The drawing under review shows one solid part. Ordinate dimensions are in mm from its lowest x, y, z. A direction names the side the tool comes from. Coordinates: 2 decimals unless noted, no trailing zeros. Write each loop counter-clockwise with the first axis right and the second up, starting at its lowest first coordinate (ties: lowest second). Pieces come first, ordered by that corner, then holes. Notation, with made-up numbers: (24, -32.5) - (53, -32.5) arc R5 ccw to (53, -26.5) - close; hole circle Ø10 at (85, 50). An arc over 180 degrees is marked (long way). Put each result on its own line as item: value. Start each with the question number.
Item 1: Mouldability with a two-part tool opening along Y and no side actions: class the marked faces 1, 2 and 3 as pulls with the +Y half, pulls with the -Y half, needs draft (parallel to the pull), parting line crosses it, or undercut.
Item 2: Consider section A-A on x = 77.5. Give the boundary of the cut face in (y, z).
Item 3: Machinability: for the marked faces 4 and 5, which of the approach directions +Z, -Z, +X, -X, +Y, -Y give a long, thin tool a straight path to every point of the face, cutting with its end or side? Answer none if there is none.
Item 4: To check wall thickness, follow L1, parallel to Y at x = 35.5, z = 16.5; L2, parallel to Z at x = 56.2, y = 2.1; L3, parallel to X at y = 10, z = 32.5. State the ranges of each line that lie inside material, in increasing order. Write a range as [from, to].
Item 5: Consider section D-D on z = 47.5. Give the boundary of the cut face in (x, y), then the cut area to 3 significant figures.
Item 6: Consider section C-C on x = 56.2. Give the boundary of the cut face in (y, z), then the cut area to 3 significant figures.
Item 7: For pin 1 (12 mm diameter, centred on y = 6, z = 38, fed in from +X); pin 2 (11 mm diameter, centred on x = 56.2, z = 25, fed in from -Y), all flat-tipped, find the tip position at first contact; note any pin that passes through.
Item 8: Consider section B-B on z = 25. Give the boundary of the cut face in (x, y), then the cut area to 3 significant figures.
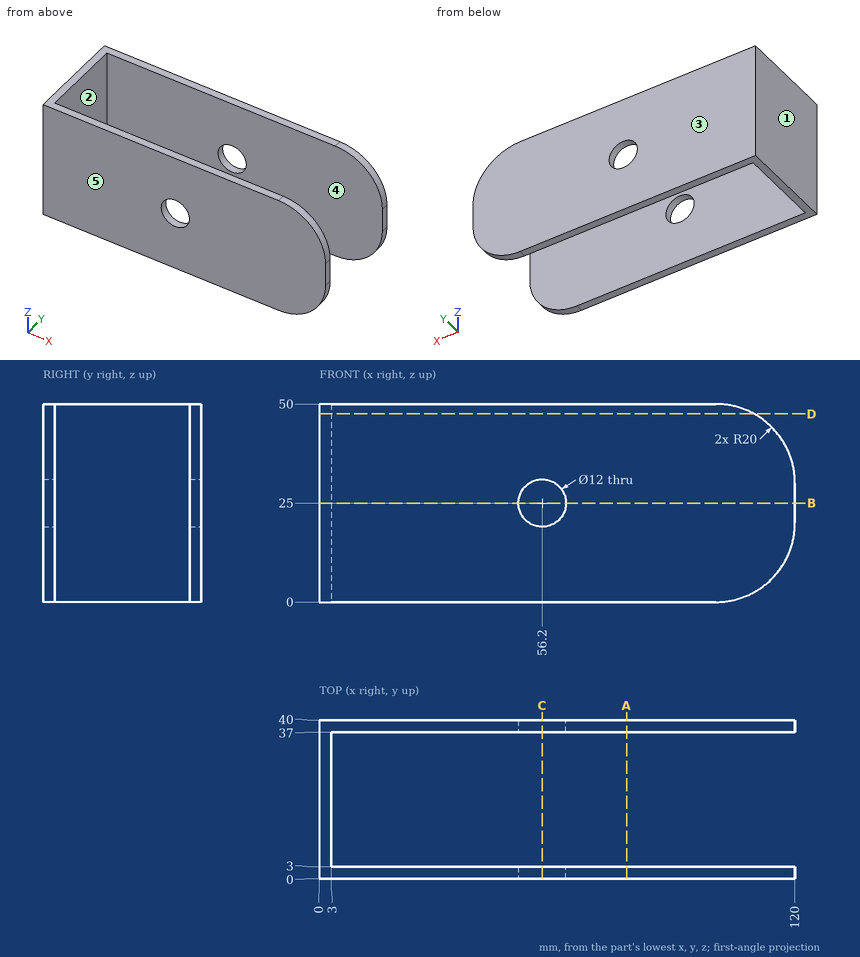
Report:
1. face 1: needs draft
1. face 2: undercut
1. face 3: pulls with the +Y half
2. outline: (0, 0) - (3, 0) - (3, 50) - (0, 50) - close; (37, 0) - (40, 0) - (40, 50) - (37, 50) - close
3. face 4: +Z, -Z, +X
3. face 5: +Z, -Z, +X, -X, -Y
4. L1: [0, 3], [37, 40]
4. L2: [0, 19], [31, 50]
4. L3: [0, 3]
5. outline: (0, 0) - (109.68, 0) - (109.68, 3) - (3, 3) - (3, 37) - (109.68, 37) - (109.68, 40) - (0, 40) - close
5. area: 760 mm²
6. outline: (0, 0) - (3, 0) - (3, 19) - (0, 19) - close; (0, 31) - (3, 31) - (3, 50) - (0, 50) - close; (37, 0) - (40, 0) - (40, 19) - (37, 19) - close; (37, 31) - (40, 31) - (40, 50) - (37, 50) - close
6. area: 228 mm²
7. pin 1: x = 119.8
7. pin 2: through
8. outline: (0, 0) - (50.2, 0) - (50.2, 3) - (3, 3) - (3, 37) - (50.2, 37) - (50.2, 40) - (0, 40) - close; (62.2, 0) - (120, 0) - (120, 3) - (62.2, 3) - close; (62.2, 37) - (120, 37) - (120, 40) - (62.2, 40) - close
8. area: 750 mm²
